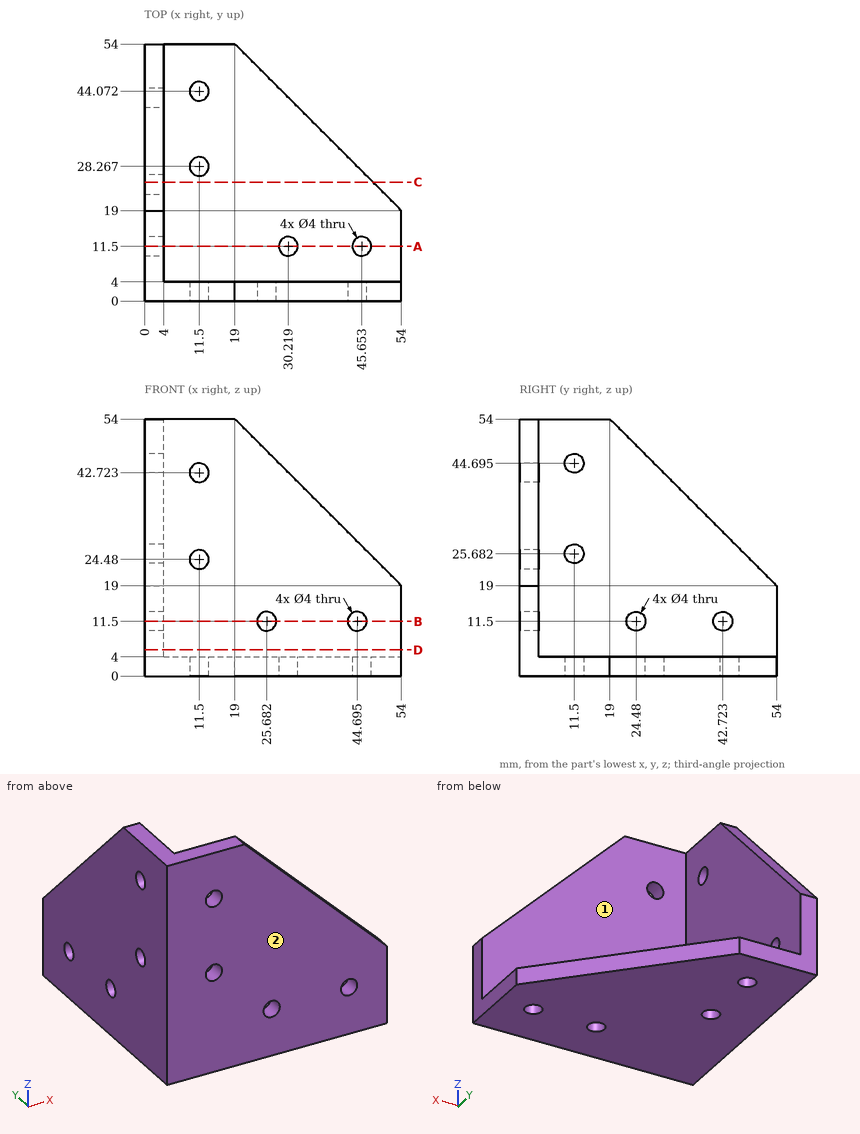
Here's the drawing with two shaded views (mm, measured from the low corner). I have some questions. A direction names the side the tool comes from. Round coordinates to 2 decimals unless told otherwise and drop trailing zeros. Order: outer loops, then holes, each group sorted by start corner. A loop starts at its lowest first (then second) coordinate and runs counter-clockwise, first axis right, second up. Notation, with made-up numbers: M -24,64 L -4,64 A25 cw -4,81 Z; hole C 12.5,21 d6. An arc over 180 degrees is marked long. Use CSV: the item, a comma, the result in double quotes.
1) I want a section at B-B (z = 11.5). List the corners of the cut face in (x, y) for me (1 decimal), then the cut area to 3 significant figures.
Taken from the geometry:
outline,"M 0,0 L 23.7,0 L 23.7,4 L 4,4 L 4,22.5 L 0,22.5 Z; M 0,26.5 L 4,26.5 L 4,40.7 L 0,40.7 Z; M 0,44.7 L 4,44.7 L 4,54 L 0,54 Z; M 27.7,0 L 42.7,0 L 42.7,4 L 27.7,4 Z; M 46.7,0 L 54,0 L 54,4 L 46.7,4 Z"
area,"352 mm^2"
2) I want a section at D-D (z = 5.5). List the corners of the cut face in (x, y) for me.
Taken from the geometry:
outline,"M 0,0 L 54,0 L 54,4 L 4,4 L 4,54 L 0,54 Z"
3) On a 3-axis mill with a long thin cutter (end or side, diameter ignored), from which of +Z, -Z, +X, -X, +Y, -Y can I reach the whole of each face in a straight line? I mean the marked faces 1 and 2. Say none if no direction works.
Taken from the geometry:
face 1,"+Z, +X, +Y"
face 2,"+Z, -Z, +X, -X, -Y"
4) I'm going to push flat-ended pins straight in: P1, Ø3, axis at x = 25.68, z = 11.5, coming from the -Y side; P2, Ø8, axis at y = 25, z = 30, coming from the -X side; P3, Ø15, axis at x = 29, y = 30.5, coming from the +Z side; P4, Ø8, axis at y = 21, z = 43, coming from the +X side. Where does each tip first touch, or does it pass through?
Taken from the geometry:
P1,"through"
P2,"x = 0"
P3,"z = 4"
P4,"x = 4"
5) I need wall thicknesses on line 1 along Z through (x, y) = (11.5, 3.1); line 2 along Y through (x, z) = (2, 11) (1 decimal); line 3 along Z through (x, y) = (44.5, 5). Which ranges of each line are inside material? Lowest first, please. Write a range as [from, to].
Taken from the geometry:
line 1,"[0, 22.48], [26.48, 40.72], [44.72, 54]"
line 2,"[0, 22.5], [26.4, 40.8], [44.7, 54]"
line 3,"[0, 4]"
6) I want a section at C-C (y = 25). List the corners of the cut face in (x, z) for me.
Taken from the geometry:
outline,"M 0,0 L 48,0 L 48,4 L 4,4 L 4,9.57 L 0,9.57 Z; M 0,13.43 L 4,13.43 L 4,48 L 0,48 Z"
7) I want a section at A-A (y = 11.5). List the corners of the cut face in (x, z) for me (1 decimal).
Taken from the geometry:
outline,"M 0,0 L 28.2,0 L 28.2,4 L 4,4 L 4,23.7 L 0,23.7 Z; M 0,27.7 L 4,27.7 L 4,42.7 L 0,42.7 Z; M 0,46.7 L 4,46.7 L 4,54 L 0,54 Z; M 32.2,0 L 43.7,0 L 43.7,4 L 32.2,4 Z; M 47.7,0 L 54,0 L 54,4 L 47.7,4 Z"
